Autodesk Inventor part; units mm, degrees
ref_plane "YZ Plane" through (0, 0, 0) normal (1, 0, 0) x (0, 1, 0)
ref_plane "XZ Plane" through (0, 0, 0) normal (0, 1, 0) x (-1, 0, 0)
ref_plane "XY Plane" through (0, 0, 0) normal (0, 0, 1) x (1, 0, 0)
sketch "Esboço1" plane through (0, 0, 0) normal (0, 1, 0) x (-1, 0, 0)
  line L0 (0, 0) -> (19.05, 0)
  line L1 (19.05, 0) -> (19.05, -19.05)
  line L2 (19.05, -19.05) -> (0, -19.05)
  line L3 (0, -19.05) -> (0, 0)
  line L4 (17.55, -17.55) -> (17.55, -1.5)
  line L5 (1.5, -1.5) -> (17.55, -1.5)
  line L6 (17.55, -17.55) -> (1.5, -17.55)
  line L7 (1.5, -1.5) -> (1.5, -17.55)
  dimension "d1" = 19.05
  dimension "d2" = 19.05
  dimension "d3" = 19.05
extrude "Extrusão1" add sketch "Esboço1" along normal blind 1000
sketch "Esboço2" plane through (-19.05, 0, -19.05) normal (0, 0, -1) x (-1, 0, 0)
  point P0 (-19.05, 0)
sketch "Esboço3" plane through (0, 0, 0) normal (0, 0, 1) x (1, 0, 0)
  line L0 (-19.05, 0) -> (0, 0)
  line L1 (0, 0) -> (-19.05, 0)
  line L2 (-9.525, 0) -> (-9.525, 480)
  circle A0 centre (-9.525, 479.5) radius 3.5
  circle A1 centre (-9.525, 520.5) radius 3.5
  dimension "d15" = 480
  dimension "d56" = 7
  dimension "d57" = 7
extrude "Extrusão2" cut sketch "Esboço3" against normal blind 20
sketch "Esboço6" plane through (0, 1000, 0) normal (0, 1, 0) x (1, 0, 0)
  line L0 (-19.05, 19.05) -> (0, 19.05)
  line L1 (0, 0) -> (-19.05, 0)
  line L2 (0, 19.05) -> (-19.05, 19.05)
  line L3 (-19.05, 19.05) -> (-19.05, 0)
  line L4 (-19.05, 0) -> (0, 0)
  line L5 (0, 0) -> (0, 19.05)
  line L6 (-17.55, 1.5) -> (-1.5, 1.5)
  line L7 (-17.55, 1.5) -> (-1.5, 1.5)
  line L8 (-1.5, 1.5) -> (-1.5, 17.55)
  line L9 (-1.5, 17.55) -> (-17.55, 17.55)
  line L10 (-17.55, 17.55) -> (-17.55, 1.5)
extrude "Extrusão5" add sketch "Esboço6" along normal blind 150
chamfer "Chanfro1" distance 0.5 angle 45 4 edges at (0, 575, 0) (-17.55, 575, -1.5) (-19.05, 575, -19.05) (0, 575, -19.05)
chamfer "Chanfro2" distance 0.5 angle 45 1 edges at (-19.05, 575, 0)
sketch "Esboço7" plane through (-0.5, 0, 0) normal (0, 0, 1) x (1, 0, 0)
  point P0 (0.5, 0)
sketch "Esboço8" plane through (-19.05, 0, -18.55) normal (-1, 0, 0) x (0, 0, 1)
  line L0 (18.55, 1150) -> (16.55, 550.0033)
  line L1 (16.55, 0) -> (16.55, 1150)
  line L2 (16.55, 550.0033) -> (16.55, 150.0033)
  line L3 (16.55, 150.0033) -> (1, 150.0033)
  line L4 (1, 0) -> (1, 1150)
  line L5 (8.775, 150.0033) -> (8.775, 190.0033)
  circle A0 centre (8.775, 190.0033) radius 3.5
  circle A1 centre (8.775, 150.0033) radius 3.5
  point P0 (18.55, 0)
  dimension "d44" = 600
  dimension "d45" = 400
  dimension "d46" = 40
  dimension "d47" = 7
  dimension "d48" = 7
extrude "Extrusão6" cut sketch "Esboço8" against normal blind 100
sketch "Esboço9" plane through (-19.05, 0, -18.55) normal (-1, 0, 0) x (0, 0, 1)
  circle A0 centre (8.775, 150.0033) radius 3.5
  line L0 (8.775, 150.0033) -> (8.775, 124.0033)
  line L1 (8.775, 124.0033) -> (55.0981, 124.0033)
  line L2 (18.55, 0) -> (-66.7734, 0)
  line L3 (55.0981, 124.0033) -> (-62.8208, 124.0033)
  line L4 (-62.8208, 124.0033) -> (-62.8208, 0)
  line L5 (-62.8208, 0) -> (55.0981, 0)
  line L6 (55.0981, 0) -> (55.0981, 124.0033)
  dimension "d51" = 26
extrude "Extrusão7" cut sketch "Esboço9" against normal blind 100 contours L1 L6 L5 L2 L4 L3
properties part number "suporte sensores 1m" material "Alumínio 6061"
Part model, mm, in its own coordinate system. A direction names the side the tool comes from. Round coordinates to 2 decimals unless told otherwise and drop trailing zeros. Write each loop counter-clockwise with the first axis right and the second up, starting at its lowest first coordinate (ties: lowest second). Pieces come first, ordered by that corner, then holes. Notation, with made-up numbers: (-0.75, 88.25) -> (48.25, 88.25) arc R16 ccw to (48.25, 111.25) -> close; hole circle Ø4 at (3.25, -9). An arc over 180 degrees is marked (long way). Return JSON: item names as keys, results as strings. Group by question number.
Q1. Mould opens along X. For faces 1 (the flat face through (-9, 630, -17.55)), 2 (the flat face through (-10, 124.003, -18)), 3 (the flat face through (0, 630, -9)) say: pulls with the +X half, pulls with the -X half, needs draft (parallel to the pull), parting line crosses it, or undercut.
Q2. Which spindle directions (+Z, -Z, +X, -X, +Y, -Y) get a long thin tool onto all of the face, cutting with end or side? Do faces 4 (the flat face through (-17.55, 630, -10)), 5 (the flat face through (-19.05, 630, -10)). Say none if no direction does.
Q3. Pin check, flat tip, straight feed: pin 1 (1.5 mm diameter, centred on x = -13.5, z = -3, fed in from +Y). Stop position of the tip, or through.
Q4. Saw through at A-A on y = 643.5. Write the cut outline in (x, z), plus the area to 3 significant figures.
Q5. Probe L1, parallel to Z at x = -10.5, y = 435; L2, parallel to X at y = 479.5, z = -18.1 (3 decimals). List the from-to ranges inside material, lowest first. Write a range as [from, to].
Answer:
{
 "1": {"face 1": "undercut", "face 2": "needs draft", "face 3": "pulls with the +X half"},
 "2": {"face 4": "+Y, -Y", "face 5": "+Z, -Z, -X, +Y, -Y"},
 "3": {"pin 1": "through"},
 "4": {"outline": "(-19.05, -18.55) -> (-18.55, -19.05) -> (-0.5, -19.05) -> (0, -18.55) -> (0, -0.5) -> (-0.5, 0) -> (-18.55, 0) -> (-19.05, -0.5) -> close; hole (-17.55, -17.55) -> (-1.5, -17.55) -> (-1.5, -1.5) -> (-17.05, -1.5) -> (-17.55, -2) -> close", "area": "105 mm2"},
 "5": {"L1": "[-19.05, -17.55], [-1.5, 0]", "L2": "[-19.05, -13.025], [-6.025, 0]"}
}
